Build history of the part. All positions in model axes, mm. A direction names the side the tool comes from. Give positions to 0.01 mm unless a question says otherwise; leave off trailing zeros. Write each loop counter-clockwise with the first axis right and the second up, starting at its lowest first coordinate (ties: lowest second). Pieces come first, ordered by that corner, then holes. Notation, with made-up numbers: (-21, 30.25) -> (28, 30.25) arc R28 ccw to (28, 49.25) -> close; hole circle Ø6 at (56, 50). An arc over 180 degrees is marked (long way). Put each result on its own line as item: value. Start each with the question number.
Item 1: Two-plate mould, pull along Z, no slides. Class faces 1 (the flat face through (0, 13, -2)), 2 (the flat face through (0, 6, -2.204)), 3 (the cylindrical face through (5.7, 4.54, 1.58)), 4 (the flat face through (0, 0, 1)): pulls with the +Z half, pulls with the -Z half, needs draft (parallel to the pull), parting line crosses it, or undercut.
Item 2: Drill centre lines: line 1 along Z through (x, y) = (-0.5, 10.75); line 2 along X through (y, z) = (3.5, 0.5); line 3 along Y through (x, z) = (-7.5, 5.75). Where is each one in solid material? Low to high.
Item 3: Slice it at A-A, the plane y = 4. List the corners of the cut face in (x, z).
Item 4: Slice it at D-D, the plane y = 1.25. List the corners of the cut face in (x, z), plus the area to 3 significant figures.
Item 5: Slice it at C-C, the plane z = 4.5. List the corners of the cut face in (x, y).
Item 6: Tool access for faces 5 (the flat face through (0, 6, 7.796)), 6 (the flat face through (2.191, -0.5, 3.8)), 7 (the flat face through (0, 6, -1.204)): list every direction of +Z, -Z, +X, -X, +Y, -Y with a clear straight run to the whole face (end or side of a thin tool).
Item 7: Flat gauge pins, fed straight in: pin 1 Ø6 at (y, z) = (4, 3.3) entering from -X; pin 2 Ø1.5 at (x, z) = (2, 5.5) entering from +Y; pin 3 Ø2.5 at (y, z) = (7, 1) entering from +X. Where does each tip first touch, or does it go through?
Item 8: Slice it at B-B, the plane x = -1.5. List the corners of the cut face in (y, z), plus the area to 3 significant figures.
Autodesk Inventor part; units mm, degrees
ref_plane "YZ Plane" through (0, 0, 0) normal (1, 0, 0) x (0, 1, 0)
ref_plane "XZ Plane" through (0, 0, 0) normal (0, 1, 0) x (-1, 0, 0)
ref_plane "XY Plane" through (0, 0, 0) normal (0, 0, 1) x (1, 0, 0)
sketch "Sketch1" plane through (0, 0, 0) normal (0, 1, 0) x (-1, 0, 0)
  line L0 (-6.1909, 7.7955) -> (5.8091, 7.7955)
  line L1 (5.8091, 7.7955) -> (5.8091, -2.2045)
  line L2 (5.8091, -2.2045) -> (-6.1909, -2.2045)
  line L3 (-6.1909, -2.2045) -> (-6.1909, 7.7955)
  point P0 (0, 0)
  dimension "d0" = 12
  dimension "d1" = 10
extrude "Extrusion1" add sketch "Sketch1" along normal blind 13
sketch "Sketch2" plane through (6.1909, 0, 7.7955) normal (1, 0, 0) x (0, 0, -1)
  line L0 (10, 0) -> (0, 0)
  line L1 (10, 0) -> (10, 13)
  line L2 (0, 0) -> (0, 13)
  circle A0 centre (4.5, 4) radius 1.8
  point P0 (7.7955, 0)
  dimension "d4" = 3.6
  dimension "d5" = 4
  dimension "d7" = 5.5
  dimension "d8" = 4.5
extrude "Extrusion2" cut sketch "Sketch2" against normal blind 13
sketch "Sketch3" plane through (0, 0, 0) normal (0, -1, 0) x (1, 0, 0)
  line L0 (6.1909, 7.7955) -> (-5.8091, 7.7955)
  line L1 (-5.8091, 7.7955) -> (-5.8091, -2.2045)
  line L2 (-5.8091, -2.2045) -> (6.1909, -2.2045)
  line L3 (6.1909, -2.2045) -> (6.1909, 7.7955)
  line L4 (-4.8091, 6.7955) -> (-4.8091, -1.2045)
  line L5 (-4.8091, -1.2045) -> (5.1909, -1.2045)
  line L6 (5.1909, -1.2045) -> (5.1909, 6.7955)
  line L7 (5.1909, 6.7955) -> (-4.8091, 6.7955)
  point P0 (0, 0)
  dimension "d11" = 1
  dimension "d12" = 1
  dimension "d14" = 1
  dimension "d15" = 1
extrude "Extrusion3" cut sketch "Sketch3" against normal blind 13 contours L7 L6 L5 L4
sketch "Sketch4" plane through (0, 0, 0) normal (0, -1, 0) x (1, 0, 0)
  line L0 (6.1909, 7.7955) -> (-5.8091, 7.7955)
  line L1 (-5.8091, 7.7955) -> (-5.8091, -2.2045)
  line L2 (-5.8091, -2.2045) -> (6.1909, -2.2045)
  line L3 (6.1909, -2.2045) -> (6.1909, 7.7955)
  line L4 (-8.8091, 8.7955) -> (-8.8091, -3.2045)
  line L5 (-8.8091, -3.2045) -> (9.1909, -3.2045)
  line L6 (9.1909, -3.2045) -> (9.1909, 8.7955)
  line L7 (9.1909, 8.7955) -> (-8.8091, 8.7955)
  point P0 (0, 0)
  dimension "d18" = 3
  dimension "d19" = 3
  dimension "d20" = 1
  dimension "d21" = 1
  dimension "d34" = 18
  dimension "d35" = 12
  dimension "d36" = 12
extrude "Extrusion4" add sketch "Sketch4" along normal blind 1 contours L3 L2 L1 L0 | L7 L6 L5 L4
sketch "Sketch5" plane through (0, -1, 0) normal (0, -1, 0) x (1, 0, 0)
  line L0 (9.1909, -3.2045) -> (9.1909, 8.7955)
  line L1 (9.1909, 8.7955) -> (-8.8091, 8.7955)
  line L2 (0.1909, 5.7955) -> (2.1909, 5.7955)
  line L3 (2.1909, 5.7955) -> (2.1909, 1.7955)
  line L4 (2.1909, 1.7955) -> (-1.8091, 1.7955)
  line L5 (-1.8091, 1.7955) -> (-1.8091, 5.7955)
  line L6 (-1.8091, 5.7955) -> (2.1909, 5.7955)
  point P0 (0, 0)
  dimension "d27" = 2
  dimension "d28" = 4
  dimension "d29" = 4
  dimension "d30" = 3
  dimension "d31" = 9
extrude "Extrusion5" cut sketch "Sketch5" against normal blind 1
properties part number "krytymotor"
Values follow:
1. face 1: needs draft
1. face 2: pulls with the -Z half
1. face 3: undercut
1. face 4: undercut
2. line 1: -2.2 to -1.2, 6.8 to 7.8
2. line 2: -5.81 to -4.81, 5.19 to 6.19
2. line 3: -1 to 0
3. outline: (-5.81, -2.2) -> (6.19, -2.2) -> (6.19, 1.5) -> (5.19, 1.5) -> (5.19, -1.2) -> (-4.81, -1.2) -> (-4.81, 1.5) -> (-5.81, 1.5) -> close; (-5.81, 5.1) -> (-4.81, 5.1) -> (-4.81, 6.8) -> (5.19, 6.8) -> (5.19, 5.1) -> (6.19, 5.1) -> (6.19, 7.8) -> (-5.81, 7.8) -> close
4. outline: (-5.81, -2.2) -> (6.19, -2.2) -> (6.19, 7.8) -> (-5.81, 7.8) -> close; hole (-4.81, -1.2) -> (5.19, -1.2) -> (5.19, 6.8) -> (-4.81, 6.8) -> close
4. area: 40.0 mm2
5. outline: (-8.81, -1) -> (-1.81, -1) -> (-1.81, 0) -> (-4.81, 0) -> (-4.81, 2.66) -> (-5.81, 2.66) -> (-5.81, 0) -> (-8.81, 0) -> close; (-5.81, 5.34) -> (-4.81, 5.34) -> (-4.81, 13) -> (-5.81, 13) -> close; (2.19, -1) -> (9.19, -1) -> (9.19, 0) -> (6.19, 0) -> (6.19, 2.66) -> (5.19, 2.66) -> (5.19, 0) -> (2.19, 0) -> close; (5.19, 5.34) -> (6.19, 5.34) -> (6.19, 13) -> (5.19, 13) -> close
6. face 5: +Z, +X, -X, +Y
6. face 6: +Y, -Y
6. face 7: +Y
7. pin 1: x = -5.81
7. pin 2: y = 0
7. pin 3: x = 6.19
8. outline: (-1, -3.2) -> (0, -3.2) -> (0, -2.2) -> (13, -2.2) -> (13, -1.2) -> (0, -1.2) -> (0, 1.8) -> (-1, 1.8) -> close; (-1, 5.8) -> (0, 5.8) -> (0, 6.8) -> (13, 6.8) -> (13, 7.8) -> (0, 7.8) -> (0, 8.8) -> (-1, 8.8) -> close
8. area: 34.0 mm2
